Drawing for the job (mm, zero at the part's lowest x, y, z). Coordinates: 2 decimals unless noted, no trailing zeros. Loops run counter-clockwise (first coordinate to the right, second up) from the corner with the lowest first, then second, coordinate; pieces in that order, holes last. Notation, with made-up numbers: (76, 21) - (110, 21) arc R11 ccw to (110, 35) - close; hole circle Ø5 at (48, 78.5). An arc over 180 degrees is marked (long way). Put each result on its own line as item: value.
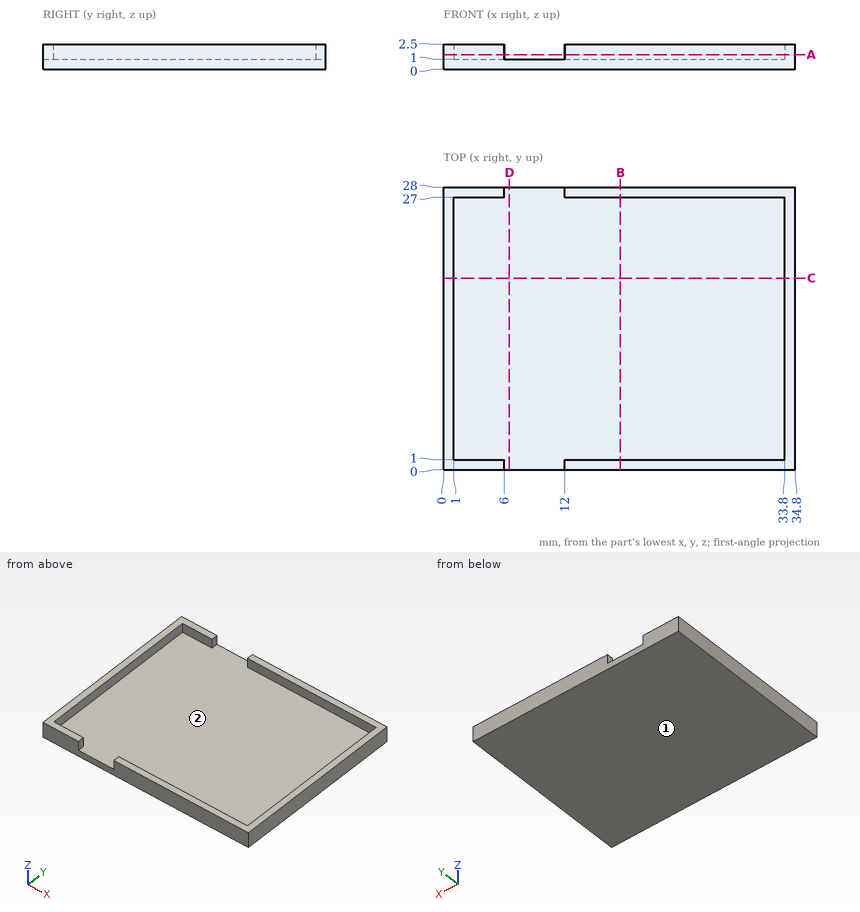
Q1. Wall check: L1, parallel to X at y = 5, z = 1.35; L2, parallel to Y at x = 16, z = 2.05; L3, parallel to Z at x = 5, y = 14.5. Give the ranges that are in metal, low to high. Write a range as from..to.
Determined:
L1: 0..1, 33.8..34.8
L2: 0..1, 27..28
L3: 0..1
Q2. Slice it at C-C, the plane y = 19. Give the cut face in (x, z), then the cut area to 3 significant figures.
Determined:
outline: (0, 0) - (34.8, 0) - (34.8, 2.5) - (33.8, 2.5) - (33.8, 1) - (1, 1) - (1, 2.5) - (0, 2.5) - close
area: 37.8 mm2
Q3. Slice it at B-B, the plane x = 17.5. Give the cut face in (y, z), then the cut area to 3 significant figures.
Determined:
outline: (0, 0) - (28, 0) - (28, 2.5) - (27, 2.5) - (27, 1) - (1, 1) - (1, 2.5) - (0, 2.5) - close
area: 31.0 mm2
Q4. Slice it at D-D, the plane x = 6.5. Give the cut face in (y, z).
Determined:
outline: (0, 0) - (28, 0) - (28, 1) - (0, 1) - close
Q5. Mould opens along Y. For the marked faces 1 and 2 say: +Y half, -Y half, draft (parallel to the pull), parting line (faces both ways), or undercut.
Determined:
face 1: draft
face 2: undercut
Q6. Slice it at A-A, the plane z = 1.45. Give the cut face in (x, y).
Determined:
outline: (0, 0) - (6, 0) - (6, 1) - (1, 1) - (1, 27) - (6, 27) - (6, 28) - (0, 28) - close; (12, 0) - (34.8, 0) - (34.8, 28) - (12, 28) - (12, 27) - (33.8, 27) - (33.8, 1) - (12, 1) - close
Q7. Pin check, flat tip, straight feed: pin 1 Ø3 at (x, y) = (15.5, 22.5) entering from +Z. Stop position of the tip, or through.
Determined:
pin 1: z = 1
